Work out the finished part from the listing and answer in its coordinate system (mm). A direction names the side the tool comes from. Give positions to 0.01 mm unless a question says otherwise; leave off trailing zeros. Write each loop counter-clockwise with the first axis right and the second up, starting at its lowest first coordinate (ties: lowest second). Pieces come first, ordered by that corner, then holes. Notation, with made-up numbers: (38, -2) -> (59, -2) arc R7 cw to (59, 10) -> close; hole circle Ø2 at (76.5, 9.25). An arc over 180 degrees is marked (long way). Write item = value, one per line. Start each with the question number.
from build123d import *

# Parameters (mm, degrees)
ESBO_O1_W                  = 40
ESBO_O1_H                  = 34
ESBO_O1_R                  = 1.5
ESBO_O1_W_2                = 22.5
ESBO_O1_H_2                = 12
RESSALTO_EXTRUS_O1_DEPTH   = 3
ESBO_O2_W                  = 40
ESBO_O2_H                  = 2.5
RESSALTO_EXTRUS_O2_DEPTH   = 30
CORTE_EXTRUS_O1_DEPTH      = 53.282720471
CORTE_EXTRUS_O1_DEPTH_BACK = 53.282720471
ESBO_O3_R                  = 3.5
FILETE1_R                  = 6
FILETE2_R                  = 2
CORTE_EXTRUS_O2_DEPTH      = 1
FILETE4_R                  = 8


with BuildPart() as part:
    # Esboço1 → Ressalto-extrusão1 (new body)
    with BuildSketch(Plane.XY):
        with Locations((-2.101648352, 0.459478022)):
            Rectangle(ESBO_O1_W, ESBO_O1_H)
        with Locations((11.648351648, 0.459478022)):
            Circle(ESBO_O1_R, mode=Mode.SUBTRACT)
        with Locations(Location((-15.851648352, 0.459478022, 0), (0, 0, 180))):
            Circle(ESBO_O1_R, mode=Mode.SUBTRACT)
        with Locations((-2.101648352, 0.459478022)):
            Rectangle(ESBO_O1_W_2, ESBO_O1_H_2, mode=Mode.SUBTRACT)
    extrude(amount=RESSALTO_EXTRUS_O1_DEPTH)

    # Esboço2 → Ressalto-extrusão2 (add)
    with BuildSketch(Plane.XY.offset(3)):
        with Locations((-2.101648352, 16.209478022)):
            Rectangle(ESBO_O2_W, ESBO_O2_H)
        with Locations((-2.101648352, -15.290521978)):
            Rectangle(ESBO_O2_W, ESBO_O2_H)
    extrude(amount=RESSALTO_EXTRUS_O2_DEPTH)

    # Esboço3 → Corte-extrusão1 (cut, two sides: drawn at the far end of the back side and taken through both)
    with BuildSketch(Plane.XZ.offset(16.540521978).offset(-CORTE_EXTRUS_O1_DEPTH_BACK)):
        with Locations(Location((11.898351648, 27, 0), (0, 0, 270))):
            Circle(ESBO_O3_R)
        Polygon((-22.101648352, 3), (7.898351648, 33), (-22.101648352, 33), align=None)
    extrude(amount=CORTE_EXTRUS_O1_DEPTH + CORTE_EXTRUS_O1_DEPTH_BACK, mode=Mode.SUBTRACT)

    # Filete1
    filete1_edges = [part.edges().sort_by_distance(p)[0] for p in [
        (17.898351648, 16.209478022, 33),
        (17.898351648, -15.290521978, 33),
    ]]
    fillet(filete1_edges, radius=FILETE1_R)

    # Filete2
    filete2_edges = [part.edges().sort_by_distance(p)[0] for p in [
        (-2.101648352, 14.959478022, 3),
        (-2.101648352, -14.040521978, 3),
    ]]
    fillet(filete2_edges, radius=FILETE2_R)

    # Esboço4 → Corte-extrusão2 (cut)
    with BuildSketch(Plane.XZ.offset(16.540521978)):
        Polygon((8.398351648, 27), (-2.157894846, 16.343280995), (1.213419281, 13.003751923), (11.621565934, 23.510961498), align=None)
    extrude(amount=-CORTE_EXTRUS_O2_DEPTH, mode=Mode.SUBTRACT)

    # Filete4
    filete4_edges = [part.edges().sort_by_distance(p)[0] for p in [
        (7.898351648, -15.290521978, 33),
        (7.898351648, 16.209478022, 33),
    ]]
    fillet(filete4_edges, radius=FILETE4_R)


solid = part.part
(1) This flat-tipped pin is pushed along its axis until it touches: pin 1 (1.8 mm diameter, centred on x = 11.65, y = 0.46, fed in from +Z). Where does it stop, or does it pass through?
(2) A cutting plane is placed at D-D, the plane x = 3.5. Write down the section's boundary in (y, z).
(3) Determine the mould class of faces 4 (the flat face through (-2, -5.541, 1)), 5 (the flat face through (2, 17.459, 13)), 6 (the flat face through (-8.5, 16.2, 16.6)) for opening direction Y: pulls with the +Y half, pulls with the -Y half, needs draft (parallel to the pull), parting line crosses it, or undercut.
(4) A cutting plane is placed at A-A, the plane y = -3. Write down the section's boundary in (x, z), then the cut area to 3 significant figures.
(5) For faces 1 (the flat face through (6.34, -16.05, 18.18)), 2 (the flat face through (-13.352, 0, 1)), 3 (the cylindrical face through (-1.82, 14.39, 3.6)), determine the directions among +Z, -Z, +X, -X, +Y, -Y from which every point of the face is accessible in a straight line to the end or side of a thin tool.
(6) A cutting plane is placed at C-C, the plane z = 26.5. Write down the section's boundary in (x, y), then the cut area to 3 significant figures.
(7) A cutting plane is placed at B-B, the plane z = 8.5. Write down the section's boundary in (x, y).
(8) Find the intervals of material crossed by line 1 along Y through (x, z) = (-3, 7.5); line 2 along Y through (x, z) = (0, 17); line 3 along Z through (x, y) = (-16.5, 5), in increasing order.
Results list:
q1.pin_1 = through
q2.outline = (-16.54, 0) -> (-5.54, 0) -> (-5.54, 3) -> (-12.04, 3) arc R2 cw to (-14.04, 5) -> (-14.04, 28.6) -> (-16.54, 28.6) -> (-16.54, 22.06) -> (-15.54, 22.06) -> (-15.54, 15.31) -> (-16.54, 15.31) -> close; (6.46, 0) -> (17.46, 0) -> (17.46, 28.6) -> (14.96, 28.6) -> (14.96, 5) arc R2 cw to (12.96, 3) -> (6.46, 3) -> close
q3.face_4 = undercut
q3.face_5 = pulls with the +Y half
q3.face_6 = needs draft
q4.outline = (-22.1, 0) -> (-13.35, 0) -> (-13.35, 3) -> (-22.1, 3) -> close; (9.15, 0) -> (17.9, 0) -> (17.9, 3) -> (9.15, 3) -> close
q4.area = 52.5 mm²
q5.face_1 = -Y
q5.face_2 = +Z, -Z
q5.face_3 = +Z, +X, -X
q6.outline = (1.4, -16.54) -> (7.9, -16.54) -> (7.9, -15.54) -> (8.43, -15.54) -> (8.43, -14.04) -> (1.4, -14.04) -> close; (1.4, 14.96) -> (8.43, 14.96) -> (8.43, 17.46) -> (1.4, 17.46) -> close; (15.36, -16.54) -> (17.9, -16.54) -> (17.9, -14.04) -> (15.36, -14.04) -> close; (15.36, 14.96) -> (17.9, 14.96) -> (17.9, 17.46) -> (15.36, 17.46) -> close
q6.area = 47.3 mm²
q7.outline = (-16.6, -16.54) -> (17.9, -16.54) -> (17.9, -14.04) -> (-16.6, -14.04) -> close; (-16.6, 14.96) -> (17.9, 14.96) -> (17.9, 17.46) -> (-16.6, 17.46) -> close
q8.line_1 = -16.54 to -14.04, 14.96 to 17.46
q8.line_2 = -15.54 to -14.04, 14.96 to 17.46
q8.line_3 = 0 to 3
